from build123d import *

# Parameters (mm, degrees)
SKETCH1_W           = 540
SKETCH1_H           = 190
BOSS_EXTRUDE1_DEPTH = 5
CHAMFER1_SIZE       = 1
SKETCH2_R           = 2
CUT_EXTRUDE1_DEPTH  = 5
SKETCH3_W           = 114
SKETCH3_H           = 48
CUT_EXTRUDE2_DEPTH  = 10


with BuildPart() as part:
    # Sketch1 → Boss-Extrude1 (new body)
    with BuildSketch(Plane.XY):
        with Locations((270, 95)):
            Rectangle(SKETCH1_W, SKETCH1_H)
    extrude(amount=BOSS_EXTRUDE1_DEPTH)

    # Chamfer1
    chamfer1_edges = [part.edges().sort_by_distance(p)[0] for p in [
        (540, 95, 5),
        (270, 190, 5),
        (0, 95, 5),
        (270, 190, 0),
        (540, 95, 0),
        (270, 0, 0),
        (0, 95, 0),
        (0, 190, 2.5),
        (540, 190, 2.5),
        (540, 0, 2.5),
        (0, 0, 2.5),
        (270, 0, 5),
    ]]
    chamfer(chamfer1_edges, length=CHAMFER1_SIZE)

    # Sketch2 → Cut-Extrude1 (cut)
    with BuildSketch(Plane.XY.offset(5)):
        with Locations((525, 175)):
            Circle(SKETCH2_R)
        with Locations((525, 15)):
            Circle(SKETCH2_R)
        with Locations((15, 175)):
            Circle(SKETCH2_R)
        with Locations((15, 15)):
            Circle(SKETCH2_R)
    extrude(amount=-CUT_EXTRUDE1_DEPTH, mode=Mode.SUBTRACT)

    # Sketch3 → Cut-Extrude2 (cut)
    with BuildSketch(Plane.XY.offset(5)):
        with Locations((270, 95)):
            Rectangle(SKETCH3_W, SKETCH3_H)
    extrude(amount=-CUT_EXTRUDE2_DEPTH, mode=Mode.SUBTRACT)


solid = part.part
The listing builds one solid part. Answer for the finished solid, in the listing's coordinates (mm). Coordinates: 2 decimals unless noted, no trailing zeros. Write each loop counter-clockwise with the first axis right and the second up, starting at its lowest first coordinate (ties: lowest second). Pieces come first, ordered by that corner, then holes. Notation, with made-up numbers: (-3.5, 73) - (45.5, 73) arc R24 cw to (45.5, 106) - close; hole circle Ø7 at (6.25, 45.5). An arc over 180 degrees is marked (long way). Put each result on its own line as item: value.
1. The part is cut by section A-A on x = 273. Give the vertices of the cut face in (y, z), plus the area to 3 significant figures.
Answer sheet:
outline: (0, 1) - (1, 0) - (71, 0) - (71, 5) - (1, 5) - (0, 4) - close; (119, 0) - (189, 0) - (190, 1) - (190, 4) - (189, 5) - (119, 5) - close
area: 708 mm^2
2. The part is cut by section C-C on z = 2. Give the vertices of the cut face in (x, y), plus the area to 3 significant figures.
Answer sheet:
outline: (0, 1) - (1, 0) - (539, 0) - (540, 1) - (540, 189) - (539, 190) - (1, 190) - (0, 189) - close; hole circle Ø4 at (15, 15); hole circle Ø4 at (15, 175); hole (213, 71) - (327, 71) - (327, 119) - (213, 119) - close; hole circle Ø4 at (525, 15); hole circle Ø4 at (525, 175)
area: 97,100 mm^2
3. The part is cut by section B-B on y = 111. Give the vertices of the cut face in (x, z), plus the area to 3 significant figures.
Answer sheet:
outline: (0, 1) - (1, 0) - (213, 0) - (213, 5) - (1, 5) - (0, 4) - close; (327, 0) - (539, 0) - (540, 1) - (540, 4) - (539, 5) - (327, 5) - close
area: 2,130 mm^2
4. Find the intervals of material crossed by line 1 along Y through (x, z) = (15, 2.25); line 2 along X through (y, z) = (109.5, 1.7); line 3 along X through (y, z) = (175, 2.45), in increasing order. Write a range as from..to.
Answer sheet:
line 1: y = 0..13, 17..173, 177..190
line 2: x = 0..213, 327..540
line 3: x = 0..13, 17..523, 527..540
5. A flat-ended cylindrical pin translates along its axis: pin 1 Ø3 at (x, y) = (525, 15) entering from +Z. Find the tip coordinate at first contact, or state that the pin passes through.
Answer sheet:
pin 1: passes through
